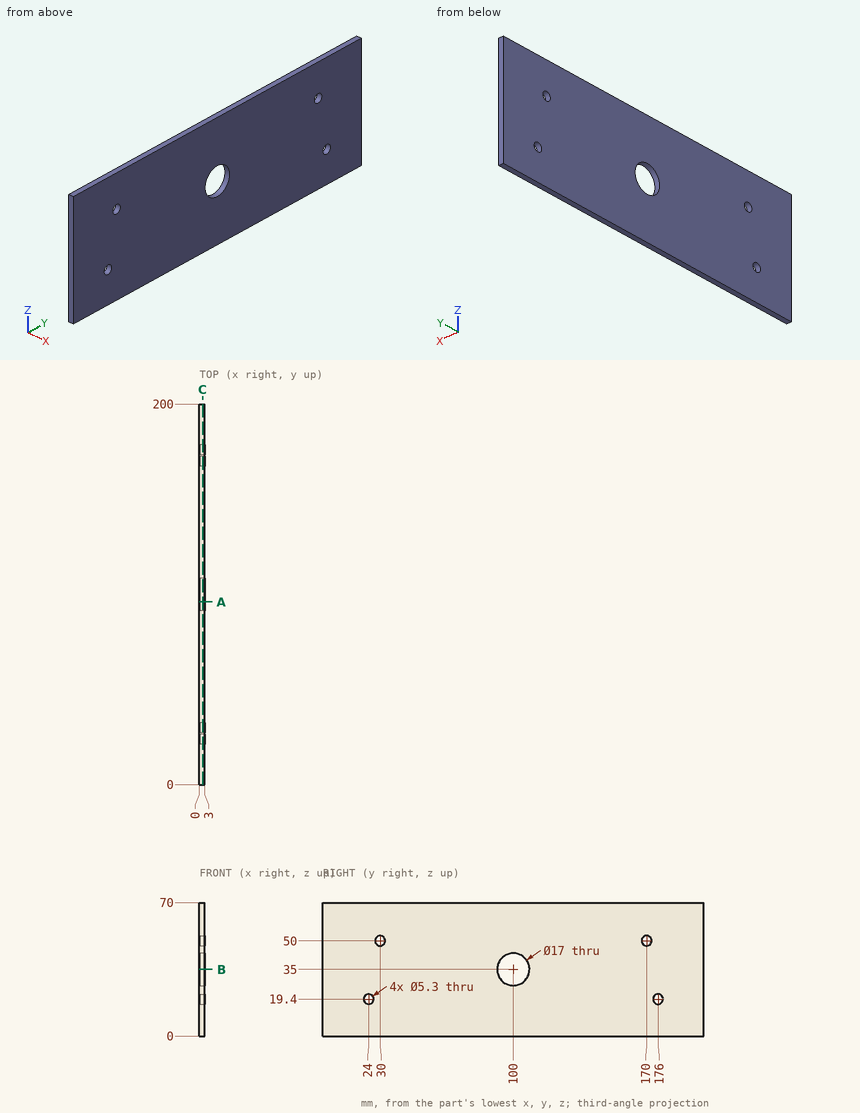
Geometry check sheet. Reference: drawing and pictorial views, mm from the part's lowest x, y, z. Round coordinates to 2 decimals unless told otherwise and drop trailing zeros. Order: outer loops, then holes, each group sorted by start corner. A loop starts at its lowest first (then second) coordinate and runs counter-clockwise, first axis right, second up. Notation, with made-up numbers: (-38.75, 20) - (4.25, 20) arc R25 ccw to (4.25, 39) - close; hole circle Ø7 at (52.5, -20). An arc over 180 degrees is marked (long way). One line per question, with ' | ' between items. Start each with the question number.
(1) Sectioned sample at B-B on z = 35. Record the cut outline in (x, y), and give its area (3 significant figures).
(2) Sectioned sample at C-C on x = 1.75. Record the cut outline in (y, z).
(3) Thickness scan on L1, parallel to Y at x = 1.6, z = 19.4; L2, parallel to Z at x = 0.7, y = 176; L3, parallel to Y at x = 0.2, z = 21.5. Record the ranges inside material, lowest first. Write a range as [from, to].
(4) Sectioned sample at A-A on y = 96. Record the cut outline in (x, z), and give its area (3 significant figures).
(5) Depth check by flat-ended pin: pin 1 Ø4 at (y, z) = (176, 19.4) entering from -X. Enter the tip coordinate at first touch or a pass-through.
Conclusion:
1) outline: (0, 0) - (3, 0) - (3, 91.5) - (0, 91.5) - close; (0, 108.5) - (3, 108.5) - (3, 200) - (0, 200) - close | area: 549 mm2
2) outline: (0, 0) - (200, 0) - (200, 70) - (0, 70) - close; hole circle Ø5.3 at (24, 19.4); hole circle Ø5.3 at (30, 50); hole circle Ø17 at (100, 35); hole circle Ø5.3 at (170, 50); hole circle Ø5.3 at (176, 19.4)
3) L1: y = [0, 21.35], [26.65, 173.35], [178.65, 200] | L2: z = [0, 16.75], [22.05, 70] | L3: y = [0, 22.38], [25.62, 174.38], [177.62, 200]
4) outline: (0, 0) - (3, 0) - (3, 27.5) - (0, 27.5) - close; (0, 42.5) - (3, 42.5) - (3, 70) - (0, 70) - close | area: 165 mm2
5) pin 1: passes through
